from build123d import *

# Parameters (mm, degrees)
SKETCH1_R           = 6.425
SKETCH1_R_2         = 4.75
BOSS_EXTRUDE1_DEPTH = 51.6
SKETCH1_3_R         = 4.75
BOSS_EXTRUDE2_DEPTH = 56.85
SKETCH1_5_R         = 15.25
SKETCH1_5_R_2       = 6.425
BOSS_EXTRUDE4_DEPTH = 49.05


with BuildPart() as part:
    # Sketch1 → Boss-Extrude1 (new body, symmetric)
    with BuildSketch(Plane(origin=(0, 0, 0), x_dir=(1, 0, 0), z_dir=(0, 1, 0))):
        Circle(SKETCH1_R)
        Circle(SKETCH1_R_2, mode=Mode.SUBTRACT)
        Circle(SKETCH1_R_2)
    extrude(amount=BOSS_EXTRUDE1_DEPTH, both=True)

    # Sketch1_3 → Boss-Extrude2 (add, symmetric)
    with BuildSketch(Plane(origin=(0, 0, 0), x_dir=(1, 0, 0), z_dir=(0, 1, 0))):
        Circle(SKETCH1_3_R)
    extrude(amount=BOSS_EXTRUDE2_DEPTH, both=True)

    # Sketch1_5 → Boss-Extrude4 (add, symmetric)
    with BuildSketch(Plane(origin=(0, 0, 0), x_dir=(1, 0, 0), z_dir=(0, 1, 0))):
        Circle(SKETCH1_5_R)
        Circle(SKETCH1_5_R_2, mode=Mode.SUBTRACT)
    extrude(amount=BOSS_EXTRUDE4_DEPTH, both=True)


solid = part.part
Here's how the part is built. I have some questions about the finished solid (model axes, mm). A direction names the side the tool comes from. Give positions to 0.01 mm unless a question says otherwise; leave off trailing zeros. Order: outer loops, then holes, each group sorted by start corner. A loop starts at its lowest first (then second) coordinate and runs counter-clockwise, first axis right, second up. Notation, with made-up numbers: (23.5, -32) -> (64.5, -32) arc R17 cw to (64.5, -4) -> close; hole circle Ø8 at (-31.75, 48). An arc over 180 degrees is marked (long way). Use a Markdown table: item, result. Add a question column.
Item 1: Imagine slicing it at D-D on z = 10. Please give me the cut outline in (x, y).
Item 2: Imagine slicing it at B-B on x = 0. Please give me the cut outline in (y, z) (3 decimals).
Item 3: If we mould it in two halves opening along Y, with no side actions, what happens to faces 1 (the face through (0, -56.85, 0)), 2 (the face through (-5.1, 50.34, 3.91)), 3 (the face through (0, 49.05, 7))? For each: pulls with the +Y half, pulls with the -Y half, needs draft (parallel to the pull), parting line crosses it, or undercut.
Item 4: For faces 4 (the face through (-1, 51.6, 5)), 5 (the face through (0, 56.85, 0)), 6 (the face through (0, -49.05, 7)), which set-ups out of +Z, -Z, +X, -X, +Y, -Y let a thin tool reach every point of the face, with its end or its side?
Item 5: I need wall thicknesses on line 1 (Y direction, x = -7.5, z = -1); line 2 (X direction, y = -25, z = -0.5); line 3 (Y direction, x = 3.5, z = 4). Which ranges of each line are inside material? Lowest first, please.
Item 6: Imagine slicing it at C-C on y = -7.5. Please give me the cut outline in (x, z), plus the area to 3 significant figures.
Item 7: Will these pins go through, and if not, where does the flat tip stop? pin 1 (1 mm diameter, centred on x = -6, y = -20, fed in from +Z); pin 2 (8 mm diameter, centred on y = -21.5, z = -9.5, fed in from -X); pin 3 (12 mm diameter, centred on y = -32.5, z = -6.5, fed in from +X); pin 4 (15 mm diameter, centred on x = 7.5, z = 4.5, fed in from -Y).
Item 8: Imagine slicing it at A-A on z = 0. Please give me the cut outline in (x, y) (3 decimals), plus the area to 3 significant figures.
Data:
| question | item | result |
|---|---|---|
| 1 | outline | (-11.51, -49.05) -> (11.51, -49.05) -> (11.51, 49.05) -> (-11.51, 49.05) -> close |
| 2 | outline | (-56.85, -4.75) -> (-51.6, -4.75) -> (-51.6, -6.425) -> (-49.05, -6.425) -> (-49.05, -15.25) -> (49.05, -15.25) -> (49.05, -6.425) -> (51.6, -6.425) -> (51.6, -4.75) -> (56.85, -4.75) -> (56.85, 4.75) -> (51.6, 4.75) -> (51.6, 6.425) -> (49.05, 6.425) -> (49.05, 15.25) -> (-49.05, 15.25) -> (-49.05, 6.425) -> (-51.6, 6.425) -> (-51.6, 4.75) -> (-56.85, 4.75) -> close |
| 3 | face 1 | pulls with the -Y half |
| 3 | face 2 | needs draft |
| 3 | face 3 | pulls with the +Y half |
| 4 | face 4 | +Y |
| 4 | face 5 | +Z, -Z, +X, -X, +Y |
| 4 | face 6 | -Y |
| 5 | line 1 | y = -49.05 to 49.05 |
| 5 | line 2 | x = -15.24 to 15.24 |
| 5 | line 3 | y = -51.6 to 51.6 |
| 6 | outline | circle Ø30.5 at (0, 0) |
| 6 | area | 731 mm² |
| 7 | pin 1 | stops at z = 14.22 |
| 7 | pin 2 | stops at x = -14.22 |
| 7 | pin 3 | stops at x = 15.24 |
| 7 | pin 4 | stops at y = -56.85 |
| 8 | outline | (-15.25, -49.05) -> (-6.425, -49.05) -> (-6.425, -51.6) -> (-4.75, -51.6) -> (-4.75, -56.85) -> (4.75, -56.85) -> (4.75, -51.6) -> (6.425, -51.6) -> (6.425, -49.05) -> (15.25, -49.05) -> (15.25, 49.05) -> (6.425, 49.05) -> (6.425, 51.6) -> (4.75, 51.6) -> (4.75, 56.85) -> (-4.75, 56.85) -> (-4.75, 51.6) -> (-6.425, 51.6) -> (-6.425, 49.05) -> (-15.25, 49.05) -> close |
| 8 | area | 3,160 mm² |
